```python
from build123d import *

# Parameters (mm, degrees)
SKETCH_R     = 9
PAD_DEPTH    = 2
SKETCH001_R  = 8
PAD001_DEPTH = 2
SKETCH002_R  = 9
PAD002_DEPTH = 9
SKETCH003_R  = 8
PAD003_DEPTH = 8
FILLET_R     = 1.5
FILLET001_R  = 0.5
FILLET002_R  = 1.5


with BuildPart() as part:
    # Sketch → Pad (new body)
    with BuildSketch(Plane.XY):
        Circle(SKETCH_R)
    extrude(amount=-PAD_DEPTH)

    # Sketch001 (on Face3 of Pad) → Pad001 (join)
    with BuildSketch(Plane(origin=(0, 0, -2), x_dir=(1, 0, 0), z_dir=(0, 0, -1))):
        Circle(SKETCH001_R)
    extrude(amount=PAD001_DEPTH)

    # Sketch002 (on Face5 of Pad001) → Pad002 (join)
    with BuildSketch(Plane(origin=(0, 0, -4), x_dir=(1, 0, 0), z_dir=(0, 0, -1))):
        Circle(SKETCH002_R)
    extrude(amount=PAD002_DEPTH)

    # Sketch003 (on Face7 of Pad002) → Pad003 (join)
    with BuildSketch(Plane(origin=(0, 0, -13), x_dir=(1, 0, 0), z_dir=(0, 0, -1))):
        Circle(SKETCH003_R)
    extrude(amount=PAD003_DEPTH)

    # Fillet
    fillet_edges = [part.edges().sort_by_distance(p)[0] for p in [
        (-9, 0, 0),
    ]]
    fillet(fillet_edges, radius=FILLET_R)

    # Fillet001
    fillet001_edges = [part.edges().sort_by_distance(p)[0] for p in [
        (-9, 0, -4),
        (-9, 0, -13),
    ]]
    fillet(fillet001_edges, radius=FILLET001_R)

    # Fillet002
    fillet002_edges = [part.edges().sort_by_distance(p)[0] for p in [
        (-8, 0, -21),
    ]]
    fillet(fillet002_edges, radius=FILLET002_R)


solid = part.part
```
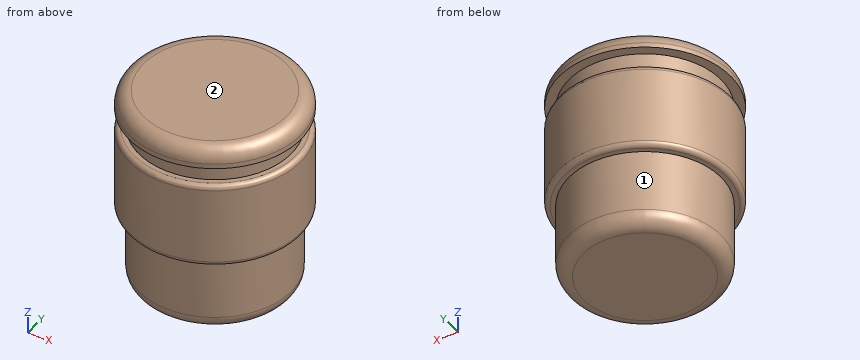
Source: CAD feature listing. Evaluate the final solid. Frame: model axes, mm. Face numbers are marked on the shaded views. A direction names the side the tool comes from. Coordinates: 2 decimals unless noted, no trailing zeros. Loops run counter-clockwise (first coordinate to the right, second up) from the corner with the lowest first, then second, coordinate; pieces in that order, holes last. Notation, with made-up numbers: M 44,69 L 67,69 A31 cw 67,96 Z; hole C 4.25,81.5 d8. An arc over 180 degrees is marked long. Put each result on its own line as item: value. Start each with the question number.
1) Reachability of the marked faces 1 and 2 from +Z, -Z, +X, -X, +Y, -Y: full face, straight path, thin tool, end or side. Return the list, or none.
2) Contact query for flat-ended pins moving along their axis: pin 1 Ø10 at (x, z) = (6.5, -14.5) entering from +Y; pin 2 Ø6 at (y, z) = (4, -12) entering from +X. Output: stop coordinate, or through.
3) Cut plane C-C on z = -11.25. Return the cut outline in (x, y).
4) Cut plane A-A on y = 0. Return the cut outline in (x, z), then the cut area to 3 significant figures.
5) Cut plane D-D on z = -19. Return the cut outline in (x, y).
6) Ray query, L1, parallel to Z at x = -7.5, y = -4.5; L2, parallel to Z at x = -7, y = 4.5; L3, parallel to Z at x = 1, y = -6.5. Return the intervals inside material, ascending. Write a range as from..to.
The answers:
1. face 1: -Z
1. face 2: +Z, +X, -X, +Y, -Y
2. pin 1: stops at y = 8.8
2. pin 2: stops at x = 8.94
3. outline: C 0,0 d18
4. outline: M -9,-12.5 A0.5 ccw -8.5,-13 L -8,-13 L -8,-19.5 A1.5 ccw -6.5,-21 L 6.5,-21 A1.5 ccw 8,-19.5 L 8,-13 L 8.5,-13 A0.5 ccw 9,-12.5 L 9,-4.5 A0.5 ccw 8.5,-4 L 8,-4 L 8,-2 L 9,-2 L 9,-1.5 A1.5 ccw 7.5,0 L -7.5,0 A1.5 ccw -9,-1.5 L -9,-2 L -8,-2 L -8,-4 L -8.5,-4 A0.5 ccw -9,-4.5 Z
4. area: 356 mm²
5. outline: C 0,0 d16
6. L1: z = -12.94..-4.06, -2..-0.67
6. L2: z = -13..-4, -2..-0.25
6. L3: z = -21..0
